from build123d import *

# Parameters (mm, degrees)
EXTRUDE_1_DEPTH     = 25
SKETCH_2_R          = 5.5
SKETCH_2_R_2        = 1.45
CUT_EXTRUDE_1_DEPTH = 10


with BuildPart() as part:
    # 草图1 → 拉伸-薄壁1 (new body)
    with BuildSketch(Plane.XY):
        Polygon((-13.990723495, 52.833651093), (-5.056846112, 37.359721559), (-0.75, 12.934383502), (-0.75, -12.934383502), (-5.056846112, -37.359721559), (-13.990723495, -52.833651093), (-12.691685389, -53.583651093), (-3.625562771, -37.880666092), (0.75, -13.065616498), (0.75, 13.065616498), (-3.625562771, 37.880666092), (-12.691685389, 53.583651093), align=None)
    extrude(amount=EXTRUDE_1_DEPTH)

    # 草图2 → 切除-拉伸1 (cut)
    with BuildSketch(Plane(origin=(0.75, 0, 0), x_dir=(0, 0, -1), z_dir=(1, 0, 0))):
        with Locations(Location((-12.5, 0, 0), (0, 0, 90))):
            Circle(SKETCH_2_R)
        with Locations(Location((-20.5, 0, 0), (0, 0, 90))):
            Circle(SKETCH_2_R_2)
        with Locations(Location((-18.156854249, 5.656854249, 0), (0, 0, 90))):
            Circle(SKETCH_2_R_2)
        with Locations(Location((-12.5, 8, 0), (0, 0, 90))):
            Circle(SKETCH_2_R_2)
        with Locations(Location((-6.843145751, 5.656854249, 0), (0, 0, 90))):
            Circle(SKETCH_2_R_2)
        with Locations(Location((-4.5, 0, 0), (0, 0, 90))):
            Circle(SKETCH_2_R_2)
        with Locations(Location((-6.843145751, -5.656854249, 0), (0, 0, 90))):
            Circle(SKETCH_2_R_2)
        with Locations(Location((-12.5, -8, 0), (0, 0, 90))):
            Circle(SKETCH_2_R_2)
        with Locations(Location((-18.156854249, -5.656854249, 0), (0, 0, 90))):
            Circle(SKETCH_2_R_2)
    extrude(amount=-CUT_EXTRUDE_1_DEPTH, mode=Mode.SUBTRACT)


solid = part.part
Geometry: final body of the model. Coordinates: model frame, mm. A direction names the side the tool comes from. Give positions to 0.01 mm unless a question says otherwise; leave off trailing zeros. Write each loop counter-clockwise with the first axis right and the second up, starting at its lowest first coordinate (ties: lowest second). Pieces come first, ordered by that corner, then holes. Notation, with made-up numbers: M -38.5,12 L -7.5,12 A20 cw -7.5,39 Z; hole C -2.5,46 d2. An arc over 180 degrees is marked long. Answer in a Markdown table with one row per item. Add a question column.
(1) Section B-B on z = 20.5. Return loops of the section in (x, y).
(2) Mould query, pull axis Y, two halves, no side actions, for faces 1 (the flat face through (-1.47, -25.65, 12.32)), 2 (the flat face through (-0.6, 0.3, 25)), 3 (the flat face through (-0.75, 0.2, 6.8)), 4 (the flat face through (-1.407, 25.299, 12.325)). Classes: +Y half, -Y half, draft (parallel to the pull), parting line (faces both ways), or undercut.
(3) Ray query, line 1 (Z direction, x = 0.45, y = 0); line 2 (Z direction, x = -0.1, y = -8); line 3 (X direction, y = 6, z = 2.75). Return the intervals inside material, ascending.
(4) First-contact query: pin 1 (8 mm diameter, centred on x = -6, z = 20, fed in from -Y); pin 2 (4 mm diameter, centred on y = -27, z = 7, fed in from -X); pin 3 (4 mm diameter, centred on y = 8, z = 12.5, fed in from -X). Flat tips, straight axial feed; report the tip coordinate or a pass-through.
(5) Section C-C on x = -6.5. Return loops of the section in (y, z).
(6) Section D-D on y = -25.5. Return loops of the section in (x, z).
(7) Reachability of faces 5 (the cylindrical face through (0, -5.8, 19.6)), 6 (the flat face through (-9.59, 45.21, 12.32)) from +Z, -Z, +X, -X, +Y, -Y: full face, straight path, thin tool, end or side. Return the list, or none.
(8) Section A-A on y = 8. Return loops of the section in (x, z).
Result set:
| question | item | result |
|---|---|---|
| 1 | outline | M -13.99,-52.83 L -12.69,-53.58 L -3.63,-37.88 L 0.75,-13.07 L 0.75,-1.45 L -0.75,-1.45 L -0.75,-12.93 L -5.06,-37.36 Z; M -13.99,52.83 L -5.06,37.36 L -0.75,12.93 L -0.75,1.45 L 0.75,1.45 L 0.75,13.07 L -3.63,37.88 L -12.69,53.58 Z |
| 2 | face 1 | -Y half |
| 2 | face 2 | draft |
| 2 | face 3 | undercut |
| 2 | face 4 | +Y half |
| 3 | line 1 | z = 0 to 3.05, 5.95 to 7, 18 to 19.05, 21.95 to 25 |
| 3 | line 2 | z = 0 to 11.05, 13.95 to 25 |
| 3 | line 3 | x = -0.75 to 0.75 |
| 4 | pin 1 | stops at y = -48.92 |
| 4 | pin 2 | stops at x = -3.58 |
| 4 | pin 3 | stops at x = -0.75 |
| 5 | outline | M -42.86,0 L -39.86,0 L -39.86,25 L -42.86,25 Z; M 39.86,0 L 42.86,0 L 42.86,25 L 39.86,25 Z |
| 6 | outline | M -2.97,0 L -1.44,0 L -1.44,25 L -2.97,25 Z |
| 7 | face 5 | +X, -X |
| 7 | face 6 | +Z, -Z, -X |
| 8 | outline | M -0.75,0 L 0.75,0 L 0.75,11.05 L -0.75,11.05 Z; M -0.75,13.95 L 0.75,13.95 L 0.75,25 L -0.75,25 Z |
